```python
from build123d import *

# Parameters (mm, degrees)
SKETCH1_W             = 43.15
SKETCH1_H             = 40
BOSS_EXTRUDE1_DEPTH   = 6
BOSS_EXTRUDE2_DEPTH   = 21
CHAMFER1_SIZE         = 11
CHAMFER1_SIZE2        = 31.45
F_5_4MM_DOWEL_HOLE1_D = 5.4
SKETCH8_R             = 4.5
BOSS_EXTRUDE3_DEPTH   = 2
F_5_4MM_DOWEL_HOLE2_D = 5.4
CUT_EXTRUDE1_DEPTH    = 44.15
FILLET1_R             = 6
FILLET2_R             = 6


with BuildPart() as part:
    # Sketch1 → Boss-Extrude1 (new body)
    with BuildSketch(Plane(origin=(0, 0, 0), x_dir=(0, 0, -1), z_dir=(1, 0, 0))):
        with Locations((21.575, 20)):
            Rectangle(SKETCH1_W, SKETCH1_H)
    extrude(amount=BOSS_EXTRUDE1_DEPTH)

    # Sketch2 → Boss-Extrude2 (add)
    with BuildSketch(Plane(origin=(0, 0, 0), x_dir=(0, 0, -1), z_dir=(1, 0, 0))):
        Polygon((-4.55, 23), (0, 23), (0, 40), (6, 40), (6, 23), (43.15, 23), (43.15, 17), (1.45, 17), (1.45, 0), (-4.55, 0), align=None)
    extrude(amount=BOSS_EXTRUDE2_DEPTH)

    # Chamfer1
    chamfer1_edges = [part.edges().sort_by_distance(p)[0] for p in [
        (21, 20, -43.15),
    ]]
    chamfer1_side = [part.faces().sort_by_distance(p)[0] for p in [
        (5.863636364, 20, -43.15),
    ]]
    chamfer(chamfer1_edges, length=CHAMFER1_SIZE, length2=CHAMFER1_SIZE2, reference=chamfer1_side[0])

    # Ø5.4mm Dowel Hole1 (through all)
    with Locations(Plane.ZY):
        with Locations((-33.15, 30), (-33.15, 10)):
            Hole(F_5_4MM_DOWEL_HOLE1_D / 2)

    # Sketch8 → Boss-Extrude3 (add)
    with BuildSketch(Plane.XY.offset(4.55)):
        with Locations((15, 10)):
            Circle(SKETCH8_R)
    extrude(amount=BOSS_EXTRUDE3_DEPTH)

    # Ø5.4mm Dowel Hole2 (through all)
    with Locations(Plane.XY.offset(6.55)):
        with Locations((15, 10)):
            Hole(F_5_4MM_DOWEL_HOLE2_D / 2)

    # Sketch11 → Cut-Extrude1 (cut, through all)
    with BuildSketch(Plane.XY):
        with BuildLine():
            Line((18.95, 36), (18.95, 30))
            ThreePointArc((18.95, 30), (17.7, 28.75), (16.45, 30))
            Line((16.45, 30), (16.45, 36))
            ThreePointArc((16.45, 36), (17.7, 37.25), (18.95, 36))
        make_face()
        with BuildLine():
            Line((9.55, 36), (9.55, 30))
            ThreePointArc((9.55, 30), (8.3, 28.75), (7.05, 30))
            Line((7.05, 30), (7.05, 36))
            ThreePointArc((7.05, 36), (8.3, 37.25), (9.55, 36))
        make_face()
    extrude(amount=-CUT_EXTRUDE1_DEPTH, mode=Mode.SUBTRACT)

    # Fillet1
    fillet1_edges = [part.edges().sort_by_distance(p)[0] for p in [
        (21, 0, 1.55),
    ]]
    fillet(fillet1_edges, radius=FILLET1_R)

    # Fillet2
    fillet2_edges = [part.edges().sort_by_distance(p)[0] for p in [
        (3, 0, -43.15),
        (3, 40, -43.15),
    ]]
    fillet(fillet2_edges, radius=FILLET2_R)


solid = part.part
```
Can you work these out from the model? Positions are in its coordinate system, mm. A direction names the side the tool comes from. Coordinates: 2 decimals unless noted, no trailing zeros. Loops run counter-clockwise (first coordinate to the right, second up) from the corner with the lowest first, then second, coordinate; pieces in that order, holes last.
Item 1: Please list where these lines run through material, in increasing order: L1, parallel to X at y = 35, z = -5; L2, parallel to Y at x = 4.7, z = -33.15; L3, parallel to Y at x = 15, z = 5.25.
Answers below:
L1: x = 0 to 7.05, 9.55 to 16.45, 18.95 to 21
L2: y = 0 to 7.3, 12.7 to 27.3, 32.7 to 40
L3: y = 5.5 to 7.3, 12.7 to 14.5
Item 2: Suppose I cut it at C-C (x = 8.3). Please give me the cut outline in (y, z).
Answers below:
outline: (0, -1.45) - (17, -1.45) - (17, -43.15) - (23, -43.15) - (23, -6) - (28.75, -6) - (28.75, 0) - (23, 0) - (23, 4.55) - (0, 4.55) - close; (37.25, -6) - (40, -6) - (40, 0) - (37.25, 0) - close
Item 3: If we mould it in two halves opening along Y, with no side actions, what happens to faces 1 (the face through (6, 9, -22)), 2 (the face through (19.289, 1.804, 1.592)), 3 (the face through (17.67, 37.25, -2.96)), 4 (the face through (10, 23, 2))? For each: released by +Y, released by -Y, zero draft, split by the parting line, or undercut.
Answers below:
face 1: zero draft
face 2: released by -Y
face 3: undercut
face 4: released by +Y
Item 4: Suppose I cut it at D-D (z = -9). Please give me the cut outline in (x, y).
Answers below:
outline: (0, 0) - (6, 0) - (6, 17) - (21, 17) - (21, 23) - (6, 23) - (6, 40) - (0, 40) - close
Item 5: Suppose I cut it at B-B (z = -3.5). Please give me the cut outline in (x, y).
Answers below:
outline: (0, 0) - (6, 0) - (6, 17) - (21, 17) - (21, 40) - (0, 40) - close; hole (7.05, 30) arc R1.25 ccw to (9.55, 30) - (9.55, 36) arc R1.25 ccw to (7.05, 36) - close; hole (16.45, 30) arc R1.25 ccw to (18.95, 30) - (18.95, 36) arc R1.25 ccw to (16.45, 36) - close
Item 6: I'm going to push flat-ended pins straight in: pin 1 (5 mm diameter, centred on y = 11.5, z = -16, fed in from +X); pin 2 (7.5 mm diameter, centred on x = 14.5, y = 28.5, fed in from -Z); pin 3 (4.5 mm diameter, centred on x = 11, z = -20, fed in from -Y); pin 4 (5 mm diameter, centred on y = 30, z = -33.15, fed in from -X). Where does each tip first touch, or does it pass through?
Answers below:
pin 1: stops at x = 6
pin 2: stops at z = -6
pin 3: stops at y = 17
pin 4: passes through
Item 7: Suppose I cut it at A-A (x = 3.75). Please give me the cut outline in (y, z), then the cut area to 3 significant figures.
Answers below:
outline: (0, -37.15) arc R6 ccw to (6, -43.15) - (34, -43.15) arc R6 ccw to (40, -37.15) - (40, 0) - (23, 0) - (23, 4.55) - (0, 4.55) - close; hole circle Ø5.4 at (10, -33.15); hole circle Ø5.4 at (30, -33.15)
area: 1,770 mm2
Item 8: Which directions (+Z, -Z, +X, -X, +Y, -Y) give clear straight access to the entire face, cutting with the end or side of a thin tool? Please do faces 5 (the face through (12, 23, -20)), 6 (the face through (8.27, 37.25, -2.96)), 7 (the face through (12, 17, -18)).
Answers below:
face 5: -Z, +X, +Y
face 6: +Z, -Z
face 7: -Z, +X, -Y
